CAD build for the part. Positions are in the model's coordinates, mm. A direction names the side the tool comes from. Round coordinates to 2 decimals unless told otherwise and drop trailing zeros. Order: outer loops, then holes, each group sorted by start corner. A loop starts at its lowest first (then second) coordinate and runs counter-clockwise, first axis right, second up.
```python
from build123d import *

# Parameters (mm, degrees)
SKETCH1_R           = 6
SKETCH1_R_2         = 7.6
BOSS_EXTRUDE1_DEPTH = 5.461
SKETCH2_W           = 12.7
SKETCH2_H           = 5.461
CUT_EXTRUDE1_DEPTH  = 6.461
SKETCH3_W           = 38.1
SKETCH3_H           = 5.08
BOSS_EXTRUDE2_DEPTH = 5.461


with BuildPart() as part:
    # Sketch1 → Boss-Extrude1 (new body)
    with BuildSketch(Plane.XY):
        Polygon((-27.903685016, 15.257451458), (27.903685016, 15.257451458), (30.1625, -16.492548542), (-30.1625, -16.492548542), align=None)
        with Locations((12.7, -3.00023153)):
            Circle(SKETCH1_R, mode=Mode.SUBTRACT)
        with Locations((-12.7, -3.00023153)):
            Circle(SKETCH1_R_2, mode=Mode.SUBTRACT)
    extrude(amount=BOSS_EXTRUDE1_DEPTH)

    # Sketch2 → Cut-Extrude1 (cut, through all)
    with BuildSketch(Plane.XY.offset(5.461)):
        with Locations((-15.875, 12.526951458)):
            Rectangle(SKETCH2_W, SKETCH2_H)
        with Locations((15.875, 12.526951458)):
            Rectangle(SKETCH2_W, SKETCH2_H)
        Polygon((-29.483716542, -6.951539225), (-28.582468475, 5.716442142), (-23.135236487, 5.328905473), (-24.036484554, -7.339075894), align=None)
        Polygon((28.582468475, 5.716442142), (29.483716542, -6.951539225), (24.036484554, -7.339075894), (23.135236487, 5.328905473), align=None)
    extrude(amount=-CUT_EXTRUDE1_DEPTH, mode=Mode.SUBTRACT)

    # Sketch3 → Boss-Extrude2 (add)
    with BuildSketch(Plane.XY.offset(5.461)):
        with Locations((0, -19.032548542)):
            Rectangle(SKETCH3_W, SKETCH3_H)
    extrude(amount=-BOSS_EXTRUDE2_DEPTH)


solid = part.part
```
1. Cut at C-C, the plane x = 12.7. Write the cut outline in (y, z).
2. Cut at D-D, the plane z = 1.8. Give the number of separate pieces and of enclosed holes in the cut face, and give its area (3 significant figures).
3. Cut at B-B, the plane y = -4.5. Write the cut outline in (x, z).
4. Pin check, flat tips, straight feed: P1, Ø1.6, axis at x = -16.5, z = 2.5, coming from the +Y side; P2, Ø1.5, axis at y = -18, z = 3.5, coming from the +X side; P3, Ø2.5, axis at y = 11.5, z = 2.5, coming from the -X side. Stop position of each tip, or through.
5. Drill centre lines: line 1 (Y direction, x = -12.7, z = 2.55); line 2 (Y direction, x = 12.7, z = 2.55); line 3 (X direction, y = -7.5, z = 2.55). Where is each one in solid material? Low to high.
6. Cut at A-A, the plane x = -12.7. Write the cut outline in (y, z), and give its area (3 significant figures).
7. Mould opens along Y. For faces 1 (the face through (-25, 15.257, 3)), 2 (the face through (-25, -16.493, 3)), 3 (the face through (-23.58, -0.92, 2.77)), 4 (the face through (-26.72, -7.15, 2.77)) say: released by +Y, released by -Y, zero draft, split by the parting line, or undercut.
8. Tool access for faces 5 (the face through (25.82, 5.52, 2.77)), 6 (the face through (-25.897, 5.525, 2.769)), 7 (the face through (-22.225, 12, 3)): list every direction of +Z, -Z, +X, -X, +Y, -Y with a clear straight run to the whole face (end or side of a thin tool).
Outcome:
1. outline: (-21.57, 0) - (-9, 0) - (-9, 5.46) - (-21.57, 5.46) - close; (3, 0) - (9.8, 0) - (9.8, 5.46) - (3, 5.46) - close
2. separate pieces: 1
2. enclosed holes: 2
2. area: 1,470 mm2
3. outline: (-23.83, 0) - (-20.15, 0) - (-20.15, 5.46) - (-23.83, 5.46) - close; (-5.25, 0) - (6.89, 0) - (6.89, 5.46) - (-5.25, 5.46) - close; (18.51, 0) - (23.83, 0) - (23.83, 5.46) - (18.51, 5.46) - close
4. P1: stops at y = 9.8
4. P2: stops at x = 19.05
4. P3: stops at x = -28.26
5. line 1: y = -21.57 to -10.6, 4.6 to 9.8
5. line 2: y = -21.57 to -9, 3 to 9.8
5. line 3: x = -29.52 to -18.82, -6.58 to 8.73, 16.67 to 29.52
6. outline: (-21.57, 0) - (-10.6, 0) - (-10.6, 5.46) - (-21.57, 5.46) - close; (4.6, 0) - (9.8, 0) - (9.8, 5.46) - (4.6, 5.46) - close
6. area: 88.3 mm2
7. face 1: released by +Y
7. face 2: released by -Y
7. face 3: undercut
7. face 4: undercut
8. face 5: +Z, -Z, +X
8. face 6: +Z, -Z, -X
8. face 7: +Z, -Z, +Y
